```python
from build123d import *

# Parameters (mm, degrees)
SKETCH1_W           = 69
SKETCH1_H           = 30
BOSS_EXTRUDE1_DEPTH = 3


with BuildPart() as part:
    # Sketch1 → Boss-Extrude1 (new body)
    with BuildSketch(Plane.XY):
        with BuildLine():
            Line((-65, 75), (-54.5, 75))
            ThreePointArc((-54.5, 75), (-47.428932188, 77.928932188), (-44.5, 85))
            Line((-44.5, 85), (-44.5, 115))
            ThreePointArc((-44.5, 115), (-41.571067812, 122.071067812), (-34.5, 125))
            Line((-34.5, 125), (34.5, 125))
            ThreePointArc((34.5, 125), (41.571067812, 122.071067812), (44.5, 115))
            Line((44.5, 115), (44.5, 85))
            ThreePointArc((44.5, 85), (47.428932188, 77.928932188), (54.5, 75))
            Line((54.5, 75), (65, 75))
            Line((65, 75), (65, -75))
            Line((65, -75), (-65, -75))
            Line((-65, -75), (-65, 75))
        make_face()
        with Locations((0, 100)):
            Rectangle(SKETCH1_W, SKETCH1_H, mode=Mode.SUBTRACT)
    extrude(amount=BOSS_EXTRUDE1_DEPTH)


solid = part.part
```
Work out the finished part from the listing and answer in its coordinate system (mm). Coordinates: 2 decimals unless noted, no trailing zeros. Write each loop counter-clockwise with the first axis right and the second up, starting at its lowest first coordinate (ties: lowest second). Pieces come first, ordered by that corner, then holes. Notation, with made-up numbers: (-6, -37.75) - (31, -37.75) arc R23 cw to (31, -7.75) - close; hole circle Ø6 at (4, 65). An arc over 180 degrees is marked (long way). Answer as a JSON object with one key per item and string values.
Q1. Find section C-C (z = 1.65). Write down the section's boundary in (x, y).
Results list:
{"outline": "(-65, -75) - (65, -75) - (65, 75) - (54.5, 75) arc R10 cw to (44.5, 85) - (44.5, 115) arc R10 ccw to (34.5, 125) - (-34.5, 125) arc R10 ccw to (-44.5, 115) - (-44.5, 85) arc R10 cw to (-54.5, 75) - (-65, 75) - close; hole (-34.5, 85) - (34.5, 85) - (34.5, 115) - (-34.5, 115) - close"}
Q2. Find section A-A (y = 90.5). Write down the section's boundary in (x, z), plus the area to 3 significant figures.
Results list:
{"outline": "(-44.5, 0) - (-34.5, 0) - (-34.5, 3) - (-44.5, 3) - close; (34.5, 0) - (44.5, 0) - (44.5, 3) - (34.5, 3) - close", "area": "60.0 mm^2"}
Q3. Given pin 1 Ø1.5 at (y, z) = (103, 2) entering from +X; pin 2 Ø1.5 at (y, z) = (93.5, 2) entering from -X, each flat-ended and moving along its own axis, determine where each tip first touches the part or whether it passes through.
Results list:
{"pin 1": "stops at x = 44.5", "pin 2": "stops at x = -44.5"}
Q4. Consider L1, parallel to Y at x = 32, z = 0.3; L2, parallel to X at y = 93, z = 1.25; L3, parallel to X at y = 115.5, z = 0.8. Determine where each line is inside the solid, lowest interval first. Write a range as from..to.
Results list:
{"L1": "y = -75..85, 115..125", "L2": "x = -44.5..-34.5, 34.5..44.5", "L3": "x = -44.49..44.49"}
Q5. Find section B-B (x = 20.5). Write down the section's boundary in (y, z).
Results list:
{"outline": "(-75, 0) - (85, 0) - (85, 3) - (-75, 3) - close; (115, 0) - (125, 0) - (125, 3) - (115, 3) - close"}
